Input: part model. Units: mm. Frame: model coordinates. Face numbers are marked on the shaded views. A direction names the side the tool comes from. Give positions to 0.01 mm unless a question says otherwise; leave off trailing zeros. Write each loop counter-clockwise with the first axis right and the second up, starting at its lowest first coordinate (ties: lowest second). Pieces come first, ordered by that corner, then holes. Notation, with made-up numbers: (-40, -15) - (-5, -15) arc R19 ccw to (-5, 13) - close; hole circle Ø7 at (29.25, 64). An arc over 180 degrees is marked (long way). Answer as CSV lines item,"result".
```python
from build123d import *

# Parameters (mm, degrees)
SKETCH_2_W          = 27.8
SKETCH_2_H          = 20
EXTRUDE_1_DEPTH     = 3.3
EXTRUDE_2_DEPTH     = 24.5
CUT_EXTRUDE_1_DEPTH = 24.8
CUT_EXTRUDE_2_DEPTH = 24.8
CUT_EXTRUDE_3_DEPTH = 24.8


with BuildPart() as part:
    # 草图2 → 凸台-拉伸1 (new body)
    with BuildSketch(Plane(origin=(0, 0, 0), x_dir=(1, 0, 0), z_dir=(0, 1, 0))):
        Rectangle(SKETCH_2_W, SKETCH_2_H)
    extrude(amount=EXTRUDE_1_DEPTH)

    # 草图4 → 凸台-拉伸2 (add)
    with BuildSketch(Plane(origin=(0, 3.3, 0), x_dir=(1, 0, 0), z_dir=(0, 1, 0))):
        Polygon((-13.9, 10), (-13.9, 6.7), (10.6, 6.7), (10.6, -6.7), (-13.9, -6.7), (-13.9, -10), (13.9, -10), (13.9, 10), align=None)
    extrude(amount=EXTRUDE_2_DEPTH)

    # 草图5 → 切除-拉伸1 (cut)
    with BuildSketch(Plane.XY.offset(10)):
        Polygon((8.801548781, 27.8), (8.801548781, 25.3), (-11.4, 5.098451219), (-13.9, 5.098451219), (-13.9, 27.8), align=None)
    extrude(amount=-CUT_EXTRUDE_1_DEPTH, mode=Mode.SUBTRACT)

    # 草图6 → 切除-拉伸2 (cut)
    with BuildSketch(Plane.ZY.offset(-10.6)):
        with BuildLine():
            Line((-3.3, 20.55), (-3.3, 10.55))
            ThreePointArc((-3.3, 10.55), (0, 7.25), (3.3, 10.55))
            Line((3.3, 10.55), (3.3, 20.55))
            ThreePointArc((3.3, 20.55), (0, 23.85), (-3.3, 20.55))
        make_face()
    extrude(amount=-CUT_EXTRUDE_2_DEPTH, mode=Mode.SUBTRACT)

    # 草图7 → 切除-拉伸3 (cut)
    with BuildSketch(Plane(origin=(0, 3.3, 0), x_dir=(1, 0, 0), z_dir=(0, 1, 0))):
        with BuildLine():
            Line((3.35, 3.3), (-6.65, 3.3))
            ThreePointArc((-6.65, 3.3), (-9.95, 0), (-6.65, -3.3))
            Line((-6.65, -3.3), (3.35, -3.3))
            ThreePointArc((3.35, -3.3), (6.65, 0), (3.35, 3.3))
        make_face()
    extrude(amount=-CUT_EXTRUDE_3_DEPTH, mode=Mode.SUBTRACT)


solid = part.part
```
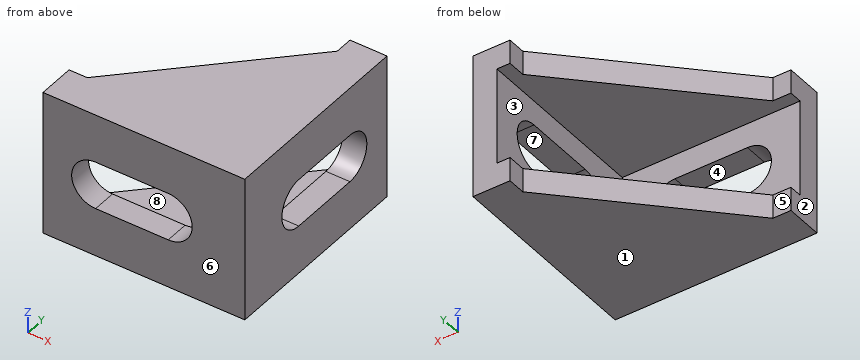
Item 1: Contact query for flat-ended pins moving along their axis: pin 1 (2 mm diameter, centred on x = -12.5, z = 9, fed in from +Y); pin 2 (6.5 mm diameter, centred on x = -3, z = 2, fed in from +Y); pin 3 (1.5 mm diameter, centred on y = 21, z = 4, fed in from -X). Output: stop coordinate, or through.
The answers:
pin 1,"y = 5.1"
pin 2,"y = 3.3"
pin 3,"x = 10.6"
Item 2: Cut plane A-A on x = 4.5. Return the cut outline in (y, z), plus the area to 3 significant figures.
The answers:
outline,"(0, -10) - (21, -10) - (21, -6.7) - (3.3, -6.7) - (3.3, -3.09) - (0, -3.09) - close; (0, 3.09) - (3.3, 3.09) - (3.3, 6.7) - (21, 6.7) - (21, 10) - (0, 10) - close"
area,"162 mm²"
Item 3: Mould query, pull axis Z, two halves, no side actions, for the marked faces 1, 2 and 3. Classes: +Z half, -Z half, draft (parallel to the pull), parting line (faces both ways), or undercut.
The answers:
face 1,"-Z half"
face 2,"draft"
face 3,"undercut"
Item 4: Cut plane D-D on x = 9.5. Return the cut outline in (y, z), plus the area to 3 significant figures.
The answers:
outline,"(0, -10) - (27.8, -10) - (27.8, -6.7) - (3.3, -6.7) - (3.3, 6.7) - (27.8, 6.7) - (27.8, 10) - (0, 10) - close"
area,"228 mm²"
Item 5: Cut plane C-C on y = 21.25. Return the cut outline in (x, z).
The answers:
outline,"(4.75, -10) - (13.9, -10) - (13.9, -3.22) - (10.6, -3.22) - (10.6, -6.7) - (4.75, -6.7) - close; (4.75, 6.7) - (10.6, 6.7) - (10.6, 3.22) - (13.9, 3.22) - (13.9, 10) - (4.75, 10) - close"
Item 6: Cut plane B-B on z = 0. Return the cut outline in (x, y).
The answers:
outline,"(-13.9, 0) - (-9.95, 0) - (-9.95, 3.3) - (-13.9, 3.3) - close; (6.65, 0) - (13.9, 0) - (13.9, 7.25) - (10.6, 7.25) - (10.6, 3.3) - (6.65, 3.3) - close; (10.6, 23.85) - (13.9, 23.85) - (13.9, 27.8) - (10.6, 27.8) - close"
Item 7: Ray query, line 1 (Z direction, x = 4.75, y = 7.75); line 2 (Z direction, x = 10.75, y = 13.75); line 3 (X direction, y = 22.5, z = -3.75). Return the intervals inside material, ascending. Write a range as from..to.
The answers:
line 1,"-10..-6.7, 6.7..10"
line 2,"-10..-3.3, 3.3..10"
line 3,"10.6..13.9"
Item 8: Reachability of the marked faces 4, 5, 6, 7 and 8 from +Z, -Z, +X, -X, +Y, -Y: full face, straight path, thin tool, end or side. Return the list, or none.
The answers:
face 4,"+Y, -Y"
face 5,"+Z, -Z, -X, +Y"
face 6,"+Z, -Z, +X, -X, -Y"
face 7,"+X, -X"
face 8,"-X, +Y"
